Model file for the job. Use its own axes, mm. Give positions to 0.01 mm unless a question says otherwise; leave off trailing zeros. Order: outer loops, then holes, each group sorted by start corner. A loop starts at its lowest first (then second) coordinate and runs counter-clockwise, first axis right, second up. Notation, with made-up numbers: (60.25, -32.5) - (98.25, -32.5) arc R27 cw to (98.25, 0.5) - close; hole circle Ø9 at (-34.75, 39.25). An arc over 180 degrees is marked (long way). Return JSON: item names as keys, results as strings. Group by question number.
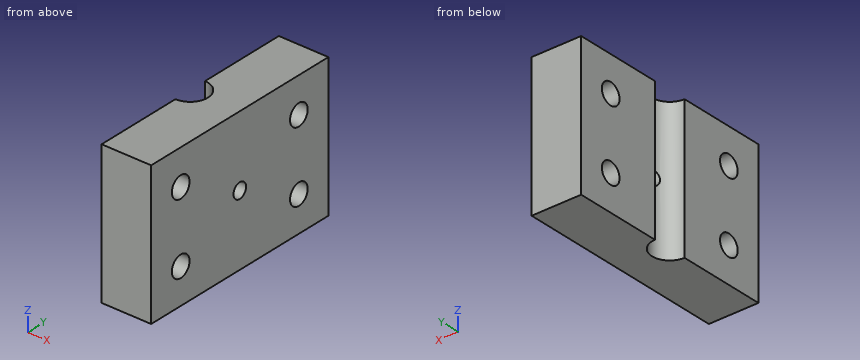
from build123d import *

# Parameters (mm, degrees)
SKETCH1_W             = 8.89
SKETCH1_H             = 25.4
BOSS_EXTRUDE1_DEPTH   = 12.7
SKETCH2_R             = 3.175
CUT_EXTRUDE1_DEPTH    = 25.4
F_6_CLEARANCE_HOLE2_D = 3.7973
F_6_32_TAPPED_HOLE1_D = 2.7051
MIRROR1_START         = -4.445
MIRROR1_OUTLINE_W     = 12.699886484
MIRROR1_OUTLINE_H     = 25.4
MIRROR1_OUTLINE_R     = 1.89865
MIRROR1_DEPTH         = 8.89


# Read off the part's stored shape, not the designer's step: Mirror1
with BuildPart() as part:
    # Sketch1 → Boss-Extrude1 (new, symmetric)
    with BuildSketch(Plane.XY):
        Rectangle(SKETCH1_W, SKETCH1_H)
    extrude(amount=BOSS_EXTRUDE1_DEPTH, both=True)

    # Sketch2 → Cut-Extrude1 (cut)
    with BuildSketch(Plane.XY.offset(12.7)):
        with Locations((-4.445, -6.35)):
            Circle(SKETCH2_R)
    extrude(amount=-CUT_EXTRUDE1_DEPTH, mode=Mode.SUBTRACT)

    # 6 Clearance Hole2 (through all)
    with Locations(Plane(origin=(4.445, 0, 0), x_dir=(0, 0, -1), z_dir=(1, 0, 0))):
        with Locations((-6.35, 6.35), (6.35, 6.35)):
            Hole(F_6_CLEARANCE_HOLE2_D / 2)

    # 6-32 Tapped Hole1 (through all)
    with Locations(Plane(origin=(4.445, 0, 0), x_dir=(0, 0, -1), z_dir=(1, 0, 0))):
        with Locations((0, -6.35)):
            Hole(F_6_32_TAPPED_HOLE1_D / 2)

    # Mirror1 outline → Mirror1 (add)
    with BuildSketch(Plane.YZ.offset(MIRROR1_START)):
        with Locations((-19.049943242, 0)):
            Rectangle(MIRROR1_OUTLINE_W, MIRROR1_OUTLINE_H)
        with Locations((-19.049886484, -6.35)):
            Circle(MIRROR1_OUTLINE_R, mode=Mode.SUBTRACT)
        with Locations((-19.049886484, 6.35)):
            Circle(MIRROR1_OUTLINE_R, mode=Mode.SUBTRACT)
    extrude(amount=MIRROR1_DEPTH)


solid = part.part
(1) Slice it at C-C (z = -6.35). Give the cut face in (x, y) (3 decimals), and give its area (3 significant figures).
(2) Slice it at A-A (y = -6.35). Give the cut face in (x, z) (3 decimals).
(3) Drill centre lines: L1, parallel to Z at x = 3, y = -6.35; L2, parallel to Y at x = 0, z = 0; L3, parallel to Z at x = 3, y = 5. Where is each one in solid material? Low to high.
(4) Slice it at B-B (x = -3.5). Give the cut face in (y, z), and give its area (3 significant figures).
(5) Slice it at D-D (y = 6.35). Give the cut face in (x, z) (3 decimals).
Result set:
{
 "1": {"outline": "(-4.445, -25.4) - (4.445, -25.4) - (4.445, -20.949) - (-4.445, -20.949) - close; (-4.445, -17.151) - (4.445, -17.151) - (4.445, 4.451) - (-4.445, 4.451) - (-4.445, -3.175) arc R3.175 cw to (-4.445, -9.525) - close; (-4.445, 8.249) - (4.445, 8.249) - (4.445, 12.7) - (-4.445, 12.7) - close", "area": "255 mm²"},
 "2": {"outline": "(-1.27, -12.7) - (4.445, -12.7) - (4.445, -1.353) - (-1.27, -1.353) - close; (-1.27, 1.353) - (4.445, 1.353) - (4.445, 12.7) - (-1.27, 12.7) - close"},
 "3": {"L1": "z = -12.7 to -1.35, 1.35 to 12.7", "L2": "y = -25.4 to -7.7, -5 to 12.7", "L3": "z = -12.7 to -7.69, -5.01 to 5.01, 7.69 to 12.7"},
 "4": {"outline": "(-25.4, -12.7) - (-9.38, -12.7) - (-9.38, 12.7) - (-25.4, 12.7) - close; (-3.32, -12.7) - (12.7, -12.7) - (12.7, 12.7) - (-3.32, 12.7) - close; hole circle Ø3.8 at (-19.05, -6.35); hole circle Ø3.8 at (-19.05, 6.35); hole circle Ø3.8 at (6.35, -6.35); hole circle Ø3.8 at (6.35, 6.35)", "area": "768 mm²"},
 "5": {"outline": "(-4.445, -12.7) - (4.445, -12.7) - (4.445, -8.249) - (-4.445, -8.249) - close; (-4.445, -4.451) - (4.445, -4.451) - (4.445, 4.451) - (-4.445, 4.451) - close; (-4.445, 8.249) - (4.445, 8.249) - (4.445, 12.7) - (-4.445, 12.7) - close"}
}
